The listing builds one solid part. Answer for the finished solid, in the listing's coordinates (mm). A direction names the side the tool comes from. Coordinates: 2 decimals unless noted, no trailing zeros. Write each loop counter-clockwise with the first axis right and the second up, starting at its lowest first coordinate (ties: lowest second). Pieces come first, ordered by that corner, then holes. Notation, with made-up numbers: M 34.25,13.5 L 54.25,13.5 A26 ccw 54.25,31.5 Z; hole C 41.25,74 d11. An arc over 180 degrees is marked long. Write item = value, one per line. Start each with the question number.
```python
from build123d import *

# Parameters (mm, degrees)
SKETCH_1_R          = 40
SKETCH_1_R_2        = 3
EXTRUDE_1_DEPTH     = 32.5
SKETCH_3_W          = 19.6
SKETCH_3_H          = 65.5
EXTRUDE_2_DEPTH     = 39
SKETCH_4_R          = 3
CUT_EXTRUDE_2_DEPTH = 57


with BuildPart() as part:
    # 草图1 → 凸台-拉伸1 (new body)
    with BuildSketch(Plane.XY):
        Circle(SKETCH_1_R)
        with Locations((-22.273863607, 22.273863607)):
            Circle(SKETCH_1_R_2, mode=Mode.SUBTRACT)
        with Locations((22.273863607, 22.273863607)):
            Circle(SKETCH_1_R_2, mode=Mode.SUBTRACT)
        with Locations((22.273863607, -22.273863607)):
            Circle(SKETCH_1_R_2, mode=Mode.SUBTRACT)
        with Locations((-22.273863607, -22.273863607)):
            Circle(SKETCH_1_R_2, mode=Mode.SUBTRACT)
    extrude(amount=EXTRUDE_1_DEPTH)

    # 草图3 → 凸台-拉伸2 (add)
    with BuildSketch(Plane(origin=(0, 0, 0), x_dir=(0, 0, -1), z_dir=(1, 0, 0))):
        with Locations((-22.7, 32.75)):
            Rectangle(SKETCH_3_W, SKETCH_3_H)
    extrude(amount=EXTRUDE_2_DEPTH)

    # 草图4 → 切除-拉伸2 (cut)
    with BuildSketch(Plane.XY):
        with Locations((22.273863607, 22.273863607)):
            Circle(SKETCH_4_R)
    extrude(amount=CUT_EXTRUDE_2_DEPTH, mode=Mode.SUBTRACT)


solid = part.part
```
1. The part is cut by section B-B, the plane z = 23. Write down the section's boundary in (x, y), and give its area (3 significant figures).
2. The part is cut by section A-A, the plane y = 24. Write down the section's boundary in (x, z), and give its area (3 significant figures).
3. The part is cut by section D-D, the plane x = 13. Write down the section's boundary in (y, z), and give its area (3 significant figures).
4. Each of these flat-tipped pins is pushed along its axis until it touches: pin 1 (3 mm diameter, centred on y = 22.5, z = 22.5, fed in from +X); pin 2 (3 mm diameter, centred on y = -18.5, z = 27, fed in from +X); pin 3 (10 mm diameter, centred on y = 11, z = 5.5, fed in from -X). Where does it stop, or does it pass through?
5. Straight lines are drawn through the part: L1, parallel to X at y = 22, z = 18; L2, parallel to X at y = 48, z = 27; L3, parallel to Z at x = 31, y = 29.5. For each, find the intervals that lie inside material, in ascending order. Write a range as [from, to].
6. For a pull along X with two mould halves and no side action, classify faces 1 (the face through (25.135, 23.175, 16.022)), 2 (the face through (39, 38, 23)), 3 (the face through (8, 13, 32.5)) as pulls with the +X half, pulls with the -X half, needs draft (parallel to the pull), parting line crosses it, or undercut.
7. For faces 4 (the face through (24, 49, 12.9)), 5 (the face through (-24.655, -24.099, 16.022)), 6 (the face through (0, 53, 23)), determine the directions among +Z, -Z, +X, -X, +Y, -Y from which every point of the face is accessible in a straight line to the end or side of a thin tool.
8. The part is cut by section C-C, the plane y = 59.5. Write down the section's boundary in (x, z).
Solution:
q1.outline = M 0,40 A40 ccw long 39,8.89 L 39,65.5 L 0,65.5 Z; hole C -22.27,-22.27 d6; hole C -22.27,22.27 d6; hole C 22.27,-22.27 d6; hole C 22.27,22.27 d6
q1.area = 6,220 mm^2
q2.outline = M -32,0 L -24.73,0 L -24.73,32.5 L -32,32.5 Z; M -19.82,0 L 19.82,0 L 19.82,32.5 L -19.82,32.5 Z; M 24.73,0 L 32,0 L 32,12.9 L 39,12.9 L 39,32.5 L 24.73,32.5 Z
q2.area = 1,900 mm^2
q3.outline = M -37.83,0 L 37.83,0 L 37.83,12.9 L 65.5,12.9 L 65.5,32.5 L -37.83,32.5 Z
q3.area = 3,000 mm^2
q4.pin_1 = 39
q4.pin_2 = 36.21
q4.pin_3 = -39.55
q5.L1 = [-33.41, -25.26], [-19.29, 19.29], [25.26, 39]
q5.L2 = [0, 39]
q5.L3 = [12.9, 32.5]
q6.face_1 = undercut
q6.face_2 = pulls with the +X half
q6.face_3 = needs draft
q7.face_4 = -Z, +X, +Y
q7.face_5 = +Z, -Z
q7.face_6 = +Z, -Z, -X, +Y
q8.outline = M 0,12.9 L 39,12.9 L 39,32.5 L 0,32.5 Z
